```python
from build123d import *

# Parameters (mm, degrees)
ESQUISSE1_W             = 200
ESQUISSE1_H             = 80
BOSS_EXTRU_1_DEPTH      = 3
CONG_1_R                = 5
ESQUISSE2_R             = 1
ENL_V_MAT_EXTRU_1_DEPTH = 216.427481998
D_GAGEMENT_M31_D        = 3.4
D_GAGEMENT_M31_DEPTH    = 10
D_GAGEMENT_M31_TIP      = 1.021463052


with BuildPart() as part:
    # Esquisse1 → Boss.-Extru.1 (new body)
    with BuildSketch(Plane(origin=(0, 0, 0), x_dir=(1, 0, 0), z_dir=(0, 1, 0))):
        with Locations((100, 40)):
            Rectangle(ESQUISSE1_W, ESQUISSE1_H)
    extrude(amount=BOSS_EXTRU_1_DEPTH)

    # Congé1
    cong_1_edges = [part.edges().sort_by_distance(p)[0] for p in [
        (0, 1.5, -80),
        (200, 1.5, -80),
        (200, 1.5, 0),
        (0, 1.5, 0),
    ]]
    fillet(cong_1_edges, radius=CONG_1_R)

    # Esquisse2 → Enlèv. mat.-Extru.1 (cut, through all)
    with BuildSketch(Plane(origin=(0, 3, 0), x_dir=(1, 0, 0), z_dir=(0, 1, 0))):
        with Locations(Location((5, 75, 0), (0, 0, 270))):
            Circle(ESQUISSE2_R)
        with Locations(Location((195, 75, 0), (0, 0, 270))):
            Circle(ESQUISSE2_R)
        with Locations(Location((195, 5, 0), (0, 0, 270))):
            Circle(ESQUISSE2_R)
        with Locations(Location((5, 5, 0), (0, 0, 270))):
            Circle(ESQUISSE2_R)
    extrude(amount=-ENL_V_MAT_EXTRU_1_DEPTH, mode=Mode.SUBTRACT)

    # Dégagement M31
    with Locations(Plane(origin=(0, 3, 0), x_dir=(1, 0, 0), z_dir=(0, 1, 0))):
        with Locations((195, 5), (5, 5), (5, 75), (195, 75)):
            Hole(D_GAGEMENT_M31_D / 2, depth=D_GAGEMENT_M31_DEPTH)
            with Locations((0, 0, -(D_GAGEMENT_M31_DEPTH + D_GAGEMENT_M31_TIP / 2))):  # 118° drill point
                Cone(0, D_GAGEMENT_M31_D / 2, D_GAGEMENT_M31_TIP, mode=Mode.SUBTRACT)


solid = part.part
```
CAD build for the part. Positions are in the model's coordinates, mm. Give positions to 0.01 mm unless a question says otherwise; leave off trailing zeros. Put each result on its own line as item: value.
Q1. Mould opens along Z. For faces 1 (the face through (193.38, 1.48, -75.51)), 2 (the face through (99, 3, -41)), 3 (the face through (199, 2, -78)), 4 (the face through (193.43, 1.48, -4.35)) say: pulls with the +Z half, pulls with the -Z half, needs draft (parallel to the pull), parting line crosses it, or undercut.
Filled in:
face 1: undercut
face 2: needs draft
face 3: pulls with the -Z half
face 4: undercut
Q2. Flat gauge pin, fed straight in: pin 1 (2.5 mm diameter, centred on x = 5, z = -5, fed in from -Y). Where does the tip first touch, or does it go through?
Filled in:
pin 1: passes through
Q3. Probe line 1 along X through (y, z) = (1.45, -75); line 2 along Z through (x, y) = (195, 1.3). List the from-to ranges inside material, lowest first.
Filled in:
line 1: x = 0 to 3.3, 6.7 to 193.3, 196.7 to 200
line 2: z = -80 to -76.7, -73.3 to -6.7, -3.3 to 0
